For this review, take the finished solid that the model builds, in its own axes (mm). A direction names the side the tool comes from. Round coordinates to 2 decimals unless told otherwise and drop trailing zeros. Write each loop counter-clockwise with the first axis right and the second up, starting at its lowest first coordinate (ties: lowest second). Pieces come first, ordered by that corner, then holes. Notation, with made-up numbers: (-4, 89.5) -> (28, 89.5) arc R20 ccw to (28, 123.5) -> close; hole circle Ø10 at (84.5, 79.25). An arc over 180 degrees is marked (long way). Write each question's results on one line, items separated by ' | '. Start each with the question number.
Item 1: The part is to be moulded in two halves that separate along Z. For faces 1 (the flat face through (94, 9, -272.5)), 2 (the flat face through (150, 1, 1)), 3 (the flat face through (76, 1.5, -4)), say which applies: +Z half, -Z half, draft (parallel to the pull), parting line (faces both ways), or undercut.
Item 2: Clearance check with flat-ended pins moving along their axes: pin 1 (5 mm diameter, centred on x = 12.25, z = 263, fed in from -Y); pin 2 (7 mm diameter, centred on x = 140.25, z = -263, fed in from +Y). State where each tip first meets the part, or that it passes through.
Item 3: To check wall thickness, follow line 1 along X through (y, z) = (1.15, 148); line 2 along X through (y, z) = (0.65, -33); line 3 along Z through (x, y) = (116, 6.25). State the ranges of each line that lie inside material, in increasing order.
Item 4: Tool access review of faces 4 (the flat face through (94, 9, -271)), 5 (the flat face through (76, 0, 4)): name each direction out of +Z, -Z, +X, -X, +Y, -Y from which nothing blocks a thin tool from reaching the whole face with its end or side.
Item 5: Add section A-A (x = 115.5). State the section outline as (y, z) points, plus the area to 3 significant figures.
Item 6: Add section B-B (z = -180). State the section outline as (x, y) points.
Item 7: Add section C-C (x = 20). State the section outline as (y, z) points, plus the area to 3 significant figures.
from build123d import *

# Parameters (mm, degrees)
ESTRUSIONE_SOTTILE1_DEPTH = 150
SCHIZZO2_R                = 3
TAGLIO_ESTRUSIONE1_DEPTH  = 566.464410905
TAGLIO_ESTRUSIONE2_DEPTH  = 566.464410905
SCHIZZO4_R                = 3
TAGLIO_ESTRUSIONE3_DEPTH  = 10
SMUSSO1_SIZE              = 5


with BuildPart() as part:
    # Schizzo1 → Estrusione-Sottile1 (new body)
    with BuildSketch(Plane(origin=(0, 0, 0), x_dir=(0, 0, -1), z_dir=(1, 0, 0))):
        with BuildLine():
            Line((-272.5, 15), (-272.5, 3))
            ThreePointArc((-272.5, 3), (-271.621320344, 0.878679656), (-269.5, 0))
            Line((-269.5, 0), (269.5, 0))
            ThreePointArc((269.5, 0), (271.621320344, 0.878679656), (272.5, 3))
            Line((272.5, 3), (272.5, 15))
            Line((272.5, 15), (271, 15))
            Line((271, 15), (271, 3))
            ThreePointArc((271, 3), (270.560660172, 1.939339828), (269.5, 1.5))
            Line((269.5, 1.5), (-269.5, 1.5))
            ThreePointArc((-269.5, 1.5), (-270.560660172, 1.939339828), (-271, 3))
            Line((-271, 3), (-271, 15))
            Line((-271, 15), (-272.5, 15))
        make_face()
    extrude(amount=ESTRUSIONE_SOTTILE1_DEPTH)

    # Schizzo2 → Taglio-Estrusione1 (cut, through all)
    with BuildSketch(Plane.XY.offset(272.5)):
        with Locations((135, 10)):
            Circle(SCHIZZO2_R)
        with Locations((50, 10)):
            Circle(SCHIZZO2_R)
    extrude(amount=-TAGLIO_ESTRUSIONE1_DEPTH, mode=Mode.SUBTRACT)

    # Schizzo3 → Taglio-Estrusione2 (cut, through all)
    with BuildSketch(Plane.XY.offset(272.5)):
        Polygon((4.5, 1.462138633), (46.165253058, 15), (0, 15), (0, 0), (4.5, 0), align=None)
    extrude(amount=-TAGLIO_ESTRUSIONE2_DEPTH, mode=Mode.SUBTRACT)

    # Schizzo4 → Taglio-Estrusione3 (cut)
    with BuildSketch(Plane(origin=(0, 1.5, 0), x_dir=(1, 0, 0), z_dir=(0, 1, 0))):
        with Locations(Location((12.2458607, 33, 0), (0, 0, 270))):
            Circle(SCHIZZO4_R)
        with Locations(Location((12.2458607, 167, 0), (0, 0, 270))):
            Circle(SCHIZZO4_R)
        with Locations(Location((12.2458607, 263, 0), (0, 0, 270))):
            Circle(SCHIZZO4_R)
        with Locations(Location((12.2458607, -263, 0), (0, 0, 270))):
            Circle(SCHIZZO4_R)
        with Locations(Location((12.2458607, -148, 0), (0, 0, 270))):
            Circle(SCHIZZO4_R)
        with Locations(Location((64.2458607, 167, 0), (0, 0, 270))):
            Circle(SCHIZZO4_R)
        with Locations(Location((89.2458607, 52, 0), (0, 0, 270))):
            Circle(SCHIZZO4_R)
        with Locations(Location((64.2458607, -33, 0), (0, 0, 270))):
            Circle(SCHIZZO4_R)
        with Locations(Location((89.2458607, -148, 0), (0, 0, 270))):
            Circle(SCHIZZO4_R)
        with Locations(Location((64.2458607, -263, 0), (0, 0, 270))):
            Circle(SCHIZZO4_R)
        with Locations(Location((140.2458607, -167, 0), (0, 0, 270))):
            Circle(SCHIZZO4_R)
        with Locations(Location((140.2458607, -52, 0), (0, 0, 270))):
            Circle(SCHIZZO4_R)
        with Locations(Location((140.2458607, 33, 0), (0, 0, 270))):
            Circle(SCHIZZO4_R)
        with Locations(Location((140.2458607, 148, 0), (0, 0, 270))):
            Circle(SCHIZZO4_R)
        with Locations(Location((89.2458607, 263, 0), (0, 0, 270))):
            Circle(SCHIZZO4_R)
        with Locations(Location((140.2458607, 263, 0), (0, 0, 270))):
            Circle(SCHIZZO4_R)
        with Locations(Location((140.2458607, -263, 0), (0, 0, 270))):
            Circle(SCHIZZO4_R)
    extrude(amount=-TAGLIO_ESTRUSIONE3_DEPTH, mode=Mode.SUBTRACT)

    # Smusso1
    smusso1_edges = [part.edges().sort_by_distance(p)[0] for p in [
        (150, 15, -271.75),
        (150, 15, 271.75),
    ]]
    chamfer(smusso1_edges, length=SMUSSO1_SIZE)


solid = part.part
Responses:
1) face 1: -Z half | face 2: draft | face 3: undercut
2) pin 1: passes through | pin 2: stops at y = 1.5
3) line 1: x = 4.5 to 9.25, 15.25 to 86.25, 92.25 to 150 | line 2: x = 4.5 to 9.25, 15.25 to 137.25, 143.25 to 150 | line 3: z = -272.5 to -271, 271 to 272.5
4) face 4: +X, -X, +Y | face 5: +Z, -Z, +X, -X, -Y
5) outline: (0, -269.5) arc R3 ccw to (3, -272.5) -> (15, -272.5) -> (15, -271) -> (3, -271) arc R1.5 cw to (1.5, -269.5) -> (1.5, 269.5) arc R1.5 cw to (3, 271) -> (15, 271) -> (15, 272.5) -> (3, 272.5) arc R3 ccw to (0, 269.5) -> close | area: 855 mm^2
6) outline: (4.5, 0) -> (150, 0) -> (150, 1.5) -> (4.62, 1.5) -> (4.5, 1.46) -> close
7) outline: (0, -269.5) arc R3 ccw to (3, -272.5) -> (6.5, -272.5) -> (6.5, -271) -> (3, -271) arc R1.5 cw to (1.5, -269.5) -> (1.5, 269.5) arc R1.5 cw to (3, 271) -> (6.5, 271) -> (6.5, 272.5) -> (3, 272.5) arc R3 ccw to (0, 269.5) -> close | area: 830 mm^2
